CAD build for the part. Positions are in the model's coordinates, mm. A direction names the side the tool comes from. Coordinates: 2 decimals unless noted, no trailing zeros. Order: outer loops, then holes, each group sorted by start corner. A loop starts at its lowest first (then second) coordinate and runs counter-clockwise, first axis right, second up. Notation, with made-up numbers: (5, -10.5) - (57, -10.5) arc R23 cw to (57, 8.5) - close; hole circle Ø4 at (17, 30). An arc over 180 degrees is marked (long way). Use one line per item in the form item = value.
```python
from build123d import *

# Parameters (mm, degrees)
BOSS_EXTRUDE1_DEPTH     = 5
SKETCH2_W               = 30
SKETCH2_H               = 19.460287126
CUT_EXTRUDE1_DEPTH      = 11
FILLET1_R               = 5
SKETCH3_R               = 1.5
CUT_EXTRUDE2_DEPTH      = 11
SKETCH4_W               = 5
SKETCH4_H               = 26.764096408
CUT_EXTRUDE3_DEPTH      = 16
CUT_EXTRUDE3_DEPTH_BACK = 16


with BuildPart() as part:
    # Sketch1 → Boss-Extrude1 (new body, symmetric)
    with BuildSketch(Plane.XY):
        Polygon((0, -17.320508076), (15, -8.660254038), (15, 8.660254038), (0, 17.320508076), (-15, 8.660254038), (-15, -8.660254038), align=None)
    extrude(amount=BOSS_EXTRUDE1_DEPTH, both=True)

    # Sketch2 → Cut-Extrude1 (cut, through all)
    with BuildSketch(Plane.XY.offset(5)):
        with Locations((0, -9.730143563)):
            Rectangle(SKETCH2_W, SKETCH2_H)
    extrude(amount=-CUT_EXTRUDE1_DEPTH, mode=Mode.SUBTRACT)

    # Fillet1
    fillet1_edges = [part.edges().sort_by_distance(p)[0] for p in [
        (-15, 8.660254038, 0),
        (0, 17.320508076, 0),
        (15, 8.660254038, 0),
    ]]
    fillet(fillet1_edges, radius=FILLET1_R)

    # Sketch3 → Cut-Extrude2 (cut, through all)
    with BuildSketch(Plane.XY.offset(5)):
        with Locations((0, 11.547005384)):
            Circle(SKETCH3_R)
    extrude(amount=-CUT_EXTRUDE2_DEPTH, mode=Mode.SUBTRACT)

    # Sketch4 → Cut-Extrude3 (cut, two sides)
    with BuildSketch(Plane(origin=(0, 0, 0), x_dir=(0, 0, -1), z_dir=(1, 0, 0))) as cut_extrude3_sk:
        with Locations((0, 16.547005384)):
            Rectangle(SKETCH4_W, SKETCH4_H)
    extrude(amount=CUT_EXTRUDE3_DEPTH, mode=Mode.SUBTRACT)
    extrude(cut_extrude3_sk.sketch, amount=-CUT_EXTRUDE3_DEPTH_BACK, mode=Mode.SUBTRACT)


solid = part.part
```
Item 1: Cut at D-D, the plane x = -10.5. Write the cut outline in (y, z).
Derived:
outline = (0, -5) - (11.26, -5) - (11.26, -2.5) - (3.16, -2.5) - (3.16, 2.5) - (11.26, 2.5) - (11.26, 5) - (0, 5) - close
Item 2: 3-axis set-ups, long thin cutter, end or side, ignore diameter. For faces 1 (the face through (0, 3.165, 0)), 2 (the face through (-0.037, 16.547, 3.768)): which of +Z, -Z, +X, -X, +Y, -Y reach the whole face in a straight line?
Derived:
face_1 = +X, -X, +Y
face_2 = +Z, -Z, +Y
Item 3: Drill centre lines: line 1 (Y direction, x = 0, z = -4.2); line 2 (Z direction, x = 12, y = 5.25); line 3 (Y direction, x = -9.5, z = -1.5). Where is each one in solid material? Low to high. Write a range as [from, to].
Derived:
line_1 = [0, 10.05], [13.05, 16.55]
line_2 = [-5, -2.5], [2.5, 5]
line_3 = [0, 3.16]
Item 4: Cut at B-B, the plane x = 0. Write the cut outline in (y, z), plus the area to 3 significant figures.
Derived:
outline = (0, -5) - (10.05, -5) - (10.05, -2.5) - (3.16, -2.5) - (3.16, 2.5) - (10.05, 2.5) - (10.05, 5) - (0, 5) - close; (13.05, -5) - (16.55, -5) - (16.55, -2.5) - (13.05, -2.5) - close; (13.05, 2.5) - (16.55, 2.5) - (16.55, 5) - (13.05, 5) - close
area = 83.6 mm²
Item 5: Cut at C-C, the plane z = -4. Write the cut outline in (x, y), plus the area to 3 significant figures.
Derived:
outline = (-15, 0) - (15, 0) - (15, 5.77) arc R5 ccw to (12.5, 10.1) - (2.5, 15.88) arc R5 ccw to (-2.5, 15.88) - (-12.5, 10.1) arc R5 ccw to (-15, 5.77) - close; hole circle Ø3 at (0, 11.55)
area = 379 mm²
Item 6: Two-plate mould, pull along Y, no slides. Class faces 3 (the face through (-0.325, 10.083, -3.732)), 4 (the face through (-0.037, 16.547, -3.732)), 5 (the face through (0, 7, 5)): +Y half, -Y half, draft (parallel to the pull), parting line (faces both ways), or undercut.
Derived:
face_3 = undercut
face_4 = +Y half
face_5 = draft
Item 7: Drop flat-ended pins along their axis: pin 1 (6 mm diameter, centred on y = 4, z = -1, fed in from +X); pin 2 (4 mm diameter, centred on x = 1.5, z = 0, fed in from +Y); pin 3 (2 mm diameter, centred on y = 13, z = -2.5, fed in from -X); pin 4 (3 mm diameter, centred on x = 11, z = -1.5, fed in from +Y). Give the stop position or say it passes through.
Derived:
pin_1 = 15
pin_2 = 3.16
pin_3 = -9.22
pin_4 = 11.62
Item 8: Cut at A-A, the plane y = 5. Write the cut outline in (x, z), plus the area to 3 significant figures.
Derived:
outline = (-15, -5) - (15, -5) - (15, -2.5) - (-15, -2.5) - close; (-15, 2.5) - (15, 2.5) - (15, 5) - (-15, 5) - close
area = 150 mm²
